Here's how the part is built. I have some questions about the finished solid (model axes, mm). Face numbers are marked on the shaded views. A direction names the side the tool comes from. Round coordinates to 2 decimals unless told otherwise and drop trailing zeros. Order: outer loops, then holes, each group sorted by start corner. A loop starts at its lowest first (then second) coordinate and runs counter-clockwise, first axis right, second up. Notation, with made-up numbers: (53, 84.5) - (111, 84.5) arc R28 ccw to (111, 118.5) - close; hole circle Ø1 at (-32, 24). An arc over 180 degrees is marked (long way). One line per item, written item: value.
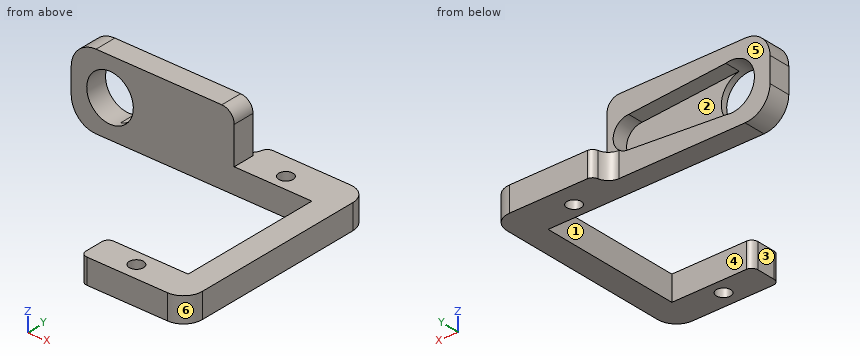
from build123d import *

# Parameters (mm, degrees)
SKETCH1_W               = 24.75
SKETCH1_H               = 12
BOSS_EXTRUDE1_DEPTH     = 3.5
SKETCH2_R               = 3.75
CUT_EXTRUDE1_DEPTH      = 15.191216474
CUT_EXTRUDE4_DEPTH      = 2.5
SKETCH5_W               = 4
SKETCH5_H               = 3.5
BOSS_EXTRUDE2_DEPTH     = 12.5
SKETCH6_W               = 4
SKETCH6_H               = 3.5
BOSS_EXTRUDE3_DEPTH     = 4
SKETCH7_W               = 4
SKETCH7_H               = 4
BOSS_EXTRUDE4_DEPTH     = 28
SKETCH8_W               = 4
SKETCH8_H               = 5
BOSS_EXTRUDE5_DEPTH     = 13
SKETCH9_W               = 16.5
SKETCH9_H               = 4
BOSS_EXTRUDE6_DEPTH     = 2.5
CUT_EXTRUDE5_DEPTH      = 42.009335827
CUT_EXTRUDE5_DEPTH_BACK = 50
SKETCH10_R              = 1.15
FILLET4_R               = 1
SKETCH13_W              = 12
SKETCH13_H              = 3.5
BOSS_EXTRUDE7_DEPTH     = 1.5
FILLET5_R               = 4
FILLET6_R               = 4
FILLET7_R               = 2
FILLET8_R               = 3
FILLET9_R               = 2


with BuildPart() as part:
    # Sketch1 → Boss-Extrude1 (new body)
    with BuildSketch(Plane(origin=(0, 0, 0), x_dir=(1, 0, 0), z_dir=(0, 1, 0))):
        Rectangle(SKETCH1_W, SKETCH1_H)
    extrude(amount=BOSS_EXTRUDE1_DEPTH)

    # Sketch2 → Cut-Extrude1 (cut, through all)
    with BuildSketch(Plane(origin=(0, 3.5, 0), x_dir=(1, 0, 0), z_dir=(0, 1, 0))):
        with Locations(Location((-7.625, 0.009358416, 0), (0, 0, 270))):
            Circle(SKETCH2_R)
    extrude(amount=-CUT_EXTRUDE1_DEPTH, mode=Mode.SUBTRACT)

    # Sketch4 → Cut-Extrude4 (cut)
    with BuildSketch(Plane(origin=(0, 3.5, 0), x_dir=(1, 0, 0), z_dir=(0, 1, 0))):
        with BuildLine():
            Line((-6.764767473, 3.659358416), (8.875, 2.509358416))
            ThreePointArc((8.875, 2.509358416), (11.375, 0.009358416), (8.875, -2.490641584))
            Line((8.875, -2.490641584), (-6.764767473, -3.640641584))
            ThreePointArc((-6.764767473, -3.640641584), (-3.875, 0.009358416), (-6.764767473, 3.659358416))
        make_face()
    extrude(amount=-CUT_EXTRUDE4_DEPTH, mode=Mode.SUBTRACT)

    # Sketch5 → Boss-Extrude2 (add)
    with BuildSketch(Plane(origin=(12.375, 0, 0), x_dir=(0, 0, -1), z_dir=(1, 0, 0))):
        with Locations((4, 1.75)):
            Rectangle(SKETCH5_W, SKETCH5_H)
    extrude(amount=BOSS_EXTRUDE2_DEPTH)

    # Sketch6 → Boss-Extrude3 (add)
    with BuildSketch(Plane(origin=(24.875, 0, 0), x_dir=(0, 0, -1), z_dir=(1, 0, 0))):
        with Locations((4, 1.75)):
            Rectangle(SKETCH6_W, SKETCH6_H)
    extrude(amount=BOSS_EXTRUDE3_DEPTH)

    # Sketch7 → Boss-Extrude4 (add)
    with BuildSketch(Plane.XZ):
        with Locations((26.875, -4)):
            Rectangle(SKETCH7_W, SKETCH7_H)
    extrude(amount=BOSS_EXTRUDE4_DEPTH)

    # Sketch8 → Boss-Extrude5 (add)
    with BuildSketch(Plane.ZY.offset(-24.875)):
        with Locations((-4, -25.5)):
            Rectangle(SKETCH8_W, SKETCH8_H)
    extrude(amount=BOSS_EXTRUDE5_DEPTH)

    # Sketch9 → Boss-Extrude6 (add)
    with BuildSketch(Plane(origin=(0, 3.5, 0), x_dir=(1, 0, 0), z_dir=(0, 1, 0))):
        with Locations((20.625, 4)):
            Rectangle(SKETCH9_W, SKETCH9_H)
    extrude(amount=BOSS_EXTRUDE6_DEPTH)

    # Sketch10 → Cut-Extrude5 (cut, two sides: drawn at the far end of the back side and taken through both)
    with BuildSketch(Plane.XY.offset(-2).offset(-CUT_EXTRUDE5_DEPTH_BACK)):
        with Locations((18.625, 2.4)):
            Circle(SKETCH10_R)
        with Locations((18.625, -25.4)):
            Circle(SKETCH10_R)
    extrude(amount=CUT_EXTRUDE5_DEPTH + CUT_EXTRUDE5_DEPTH_BACK, mode=Mode.SUBTRACT)

    # Fillet4
    fillet4_edges = [part.edges().sort_by_distance(p)[0] for p in [
        (11.875, -28, -4),
        (11.875, -23, -4),
        (12.375, 6, -4),
    ]]
    fillet(fillet4_edges, radius=FILLET4_R)

    # Sketch13 → Boss-Extrude7 (add)
    with BuildSketch(Plane.ZY.offset(12.375)):
        with Locations((0, 1.75)):
            Rectangle(SKETCH13_W, SKETCH13_H)
    extrude(amount=BOSS_EXTRUDE7_DEPTH)

    # Fillet5
    fillet5_edges = [part.edges().sort_by_distance(p)[0] for p in [
        (-13.875, 1.75, 6),
    ]]
    fillet(fillet5_edges, radius=FILLET5_R)

    # Fillet6
    fillet6_edges = [part.edges().sort_by_distance(p)[0] for p in [
        (-13.875, 1.75, -6),
    ]]
    fillet(fillet6_edges, radius=FILLET6_R)

    # Fillet7
    fillet7_edges = [part.edges().sort_by_distance(p)[0] for p in [
        (12.375, 1.75, 6),
    ]]
    fillet(fillet7_edges, radius=FILLET7_R)

    # Fillet8
    fillet8_edges = [part.edges().sort_by_distance(p)[0] for p in [
        (28.875, -28, -4),
        (28.875, 6, -4),
    ]]
    fillet(fillet8_edges, radius=FILLET8_R)

    # Fillet9
    # the kernel refuses this fillet: 2 mm, written as the material it adds along each edge
    with BuildSketch(Plane(origin=(12.375, 3.5, -6), x_dir=(0.008391726197268362, 0.9999647888458023, 0), z_dir=(0, 0, 1))) as fillet9_piece_1:
        with BuildLine():
            CenterArc((1.983498243, 1.974754399), FILLET9_R, 180.480816137, 80.405931773)
            Line((-0.016431335, 1.957970947), (-0.216424292, 1.956292601))
            Line((-0.216424292, 1.956292601), (-0.199992958, -0.001678345))
            Line((-0.199992958, -0.001678345), (0.001678345, -0.199992958))
            ThreePointArc((0.001678345, -0.199992958), (1.501625529, -0.187405368), (1.635048065, -0.19747544))
            Line((1.635048065, -0.19747544), (1.666725354, 0))
        make_face()
    extrude(amount=4)


solid = part.part
Q1. Which directions (+Z, -Z, +X, -X, +Y, -Y) give clear straight access to the entire face, cutting with the end or side of a thin tool? Please do the marked faces 1, 2 and 3.
Results list:
face 1: +Z, -Z, -X
face 2: +Y
face 3: +Z, -Z, -X, -Y
Q2. If we section it at A-A, the plane y = 2.4: Please give me the cut outline in (x, z) (3 decimals), then the cut area to 3 significant figures.
Results list:
outline: (-13.875, -2) arc R4 ccw to (-9.875, -6) - (17.475, -6) - (17.475, -2) - (12.375, -2) - (12.375, 4) arc R2 ccw to (10.375, 6) - (-9.875, 6) arc R4 ccw to (-13.875, 2) - close; (19.775, -6) - (28.875, -6) - (28.875, -2) - (19.775, -2) - close; hole (-6.765, -3.659) - (8.875, -2.509) arc R2.5 ccw to (8.875, 2.491) - (-6.765, 3.641) arc R3.75 ccw (long way) to start
area: 230 mm²
Q3. Will these pins go through, and if not, where does the flat tip stop? pin 1 (5 mm diameter, centred on y = -10.5, z = -4.5, fed in from -X) (3 decimals); pin 2 (1.5 mm diameter, centred on x = -2.5, z = -4, fed in from -Y); pin 3 (1.5 mm diameter, centred on y = -25, z = -4, fed in from -X) (3 decimals).
Results list:
pin 1: x = 24.875
pin 2: y = 0
pin 3: x = 11.875
Q4. If we section it at B-B, the plane x = 23: Please give me the cut outline in (y, z).
Results list:
outline: (-28, -6) - (-23, -6) - (-23, -2) - (-28, -2) - close; (0, -6) - (6, -6) - (6, -2) - (0, -2) - close
Q5. We'd pull the mould along Y, two halves only. Please class the marked faces 4, 5 and 6: released by +Y, released by -Y, zero draft, split by the parting line, or undercut.
Results list:
face 4: undercut
face 5: released by +Y
face 6: released by -Y
Q6. If I drill on line 1 along Y through (x, z) = (8, -2.75); line 2 along X through (y, z) = (-13.5, -4) (3 decimals); line 3 along X through (y, z) = (-25.4, -4.4) (3 decimals), over which ranges is the centre line in solid material (lowest first)?
Results list:
line 1: 0 to 3.5
line 2: 24.875 to 28.875
line 3: 11.875 to 17.475, 19.775 to 28.848
Q7. If we section it at D-D, the plane y = -10: Please give me the cut outline in (x, z) (3 decimals), then the cut area to 3 significant figures.
Results list:
outline: (24.875, -6) - (28.875, -6) - (28.875, -2) - (24.875, -2) - close
area: 16.0 mm²
Q8. If we section it at C-C, the plane z = 3: Please give me the cut outline in (x, y) (3 decimals).
Results list:
outline: (-13.748, 0) - (-9.862, 0) - (-9.862, 3.5) - (-13.748, 3.5) - close; (-5.388, 0) - (12.375, 0) - (12.375, 3.5) - (1.948, 3.5) - (1.948, 1) - (-5.388, 1) - close
